Build history of the part. All positions in model axes, mm. Face numbers are marked on the shaded views. A direction names the side the tool comes from. Give positions to 0.01 mm unless a question says otherwise; leave off trailing zeros. Loops run counter-clockwise (first coordinate to the right, second up) from the corner with the lowest first, then second, coordinate; pieces in that order, holes last. Notation, with made-up numbers: (53.5, -17.75) - (84.5, -17.75) arc R18 cw to (84.5, 14.25) - close; hole circle Ø11 at (36, 50). An arc over 180 degrees is marked (long way). Return JSON: item names as keys, results as strings. Group by question number.
1) Slice it at C-C (z = 6). List the corners of the cut face in (x, y), and give its area (3 significant figures).
2) Slice it at B-B (x = 3.5). List the corners of the cut face in (y, z).
3) Drop flat-ended pins along their axis: pin 1 (0.5 mm diameter, centred on x = 4, z = 2, fed in from -Y); pin 2 (1.5 mm diameter, centred on x = -5.5, z = 4.5, fed in from -Y); pin 3 (1.5 mm diameter, centred on x = 4, y = 6, fed in from +Z). Give the stop position or say it passes through.
4) Drill centre lines: probe 1 along Y at (x, z) = (-5, 3.5); probe 2 along Z at (x, y) = (-1.5, -2); probe 3 along X at (y, z) = (-4.25, 3.75). Where is each one in solid material? Low to high. Write a range as from..to.
5) Slice it at D-D (x = -5). List the corners of the cut face in (y, z).
6) Slice it at A-A (y = -4.5). List the corners of the cut face in (x, z).
7) 3-axis set-ups, long thin cutter, end or side, ignore diameter. For the marked faces 1, 2 and 3: which of +Z, -Z, +X, -X, +Y, -Y reach the whole face in a straight line?
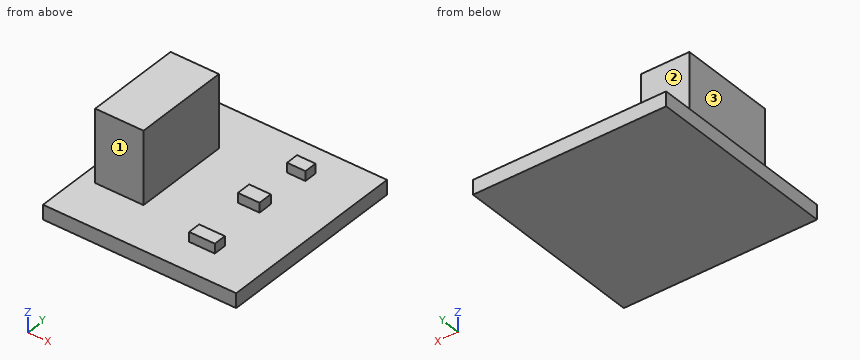
Autodesk Inventor part; units mm, degrees
ref_plane "YZ Plane" through (0, 0, 0) normal (1, 0, 0) x (0, 1, 0)
ref_plane "XZ Plane" through (0, 0, 0) normal (0, 1, 0) x (-1, 0, 0)
ref_plane "XY Plane" through (0, 0, 0) normal (0, 0, 1) x (1, 0, 0)
sketch "Sketch1" plane through (0, 0, 0) normal (0, 0, 1) x (1, 0, 0)
  line L0 (-10, -10) -> (10, -10)
  line L1 (10, -10) -> (10, 10)
  line L2 (10, 10) -> (-10, 10)
  line L3 (-10, 10) -> (-10, -10)
  line L4 (-10, -10) -> (10, 10) construction
  line L5 (10, -10) -> (-10, 10) construction
  point P0 (0, 0)
  dimension "d0" = 20
  dimension "d1" = 20
extrude "Extrusion1" add sketch "Sketch1" along normal blind 1.5
sketch "Sketch2" plane through (0, 0, 1.5) normal (0, 0, 1) x (1, 0, 0)
  line L0 (-14, 0) -> (14, 0)
  line L1 (-8.5, -5) -> (-3.5, -5)
  line L2 (-3.5, -5) -> (-3.5, 5)
  line L3 (-3.5, 5) -> (-8.5, 5)
  line L4 (-8.5, 5) -> (-8.5, -5)
  line L5 (-8.5, -5) -> (-3.5, 5) construction
  line L6 (-3.5, -5) -> (-8.5, 5) construction
  line L7 (-10, 10) -> (-10, -10)
  point P0 (0, 0)
  point P1 (-6, 0)
  dimension "d4" = 1.5
  dimension "d5" = 10
  dimension "d6" = 5
extrude "Extrusion2" add sketch "Sketch2" along normal blind 7.5
sketch "Sketch3" plane through (0, 0, 1.5) normal (0, 0, 1) x (1, 0, 0)
  line L0 (2.9488, 7.102) -> (4.8593, 7.102)
  line L1 (4.8593, 7.102) -> (4.8593, 5.773)
  line L2 (4.8593, 5.773) -> (2.9488, 5.773)
  line L3 (2.9488, 5.773) -> (2.9488, 7.102)
  line L4 (2.9488, 7.102) -> (4.8593, 5.773) construction
  line L5 (4.8593, 7.102) -> (2.9488, 5.773) construction
  line L6 (2.3673, 1.4952) -> (4.6101, 1.4952)
  line L7 (4.6101, 1.4952) -> (4.6101, 0)
  line L8 (4.6101, 0) -> (2.3673, 0)
  line L9 (2.3673, 0) -> (2.3673, 1.4952)
  line L10 (2.3673, 1.4952) -> (4.6101, 0) construction
  line L11 (4.6101, 1.4952) -> (2.3673, 0) construction
  line L12 (2.575, -5.3992) -> (5.233, -5.3992)
  line L13 (5.233, -5.3992) -> (5.233, -6.7282)
  line L14 (5.233, -6.7282) -> (2.575, -6.7282)
  line L15 (2.575, -6.7282) -> (2.575, -5.3992)
  line L16 (2.575, -5.3992) -> (5.233, -6.7282) construction
  line L17 (5.233, -5.3992) -> (2.575, -6.7282) construction
  point P0 (0, 0)
  point P1 (3.904, 6.4375)
  point P2 (3.4887, 0.7476)
  point P3 (3.904, -6.0637)
extrude "Extrusion3" add sketch "Sketch3" along normal blind 1
properties part number "sunlightsensor"
Results:
{
 "1": {"outline": "(-8.5, -5) - (-3.5, -5) - (-3.5, 5) - (-8.5, 5) - close", "area": "50.0 mm2"},
 "2": {"outline": "(-10, 0) - (10, 0) - (10, 1.5) - (7.1, 1.5) - (7.1, 2.5) - (5.77, 2.5) - (5.77, 1.5) - (1.5, 1.5) - (1.5, 2.5) - (0, 2.5) - (0, 1.5) - (-5.4, 1.5) - (-5.4, 2.5) - (-6.73, 2.5) - (-6.73, 1.5) - (-10, 1.5) - close"},
 "3": {"pin 1": "y = -6.73", "pin 2": "y = -5", "pin 3": "z = 2.5"},
 "4": {"probe 1": "-5..5", "probe 2": "0..1.5", "probe 3": "-8.5..-3.5"},
 "5": {"outline": "(-10, 0) - (10, 0) - (10, 1.5) - (5, 1.5) - (5, 9) - (-5, 9) - (-5, 1.5) - (-10, 1.5) - close"},
 "6": {"outline": "(-10, 0) - (10, 0) - (10, 1.5) - (-3.5, 1.5) - (-3.5, 9) - (-8.5, 9) - (-8.5, 1.5) - (-10, 1.5) - close"},
 "7": {"face 1": "+Z, +X, -X, -Y", "face 2": "+Z, +X, -X, +Y", "face 3": "+Z, -X, +Y, -Y"}
}
